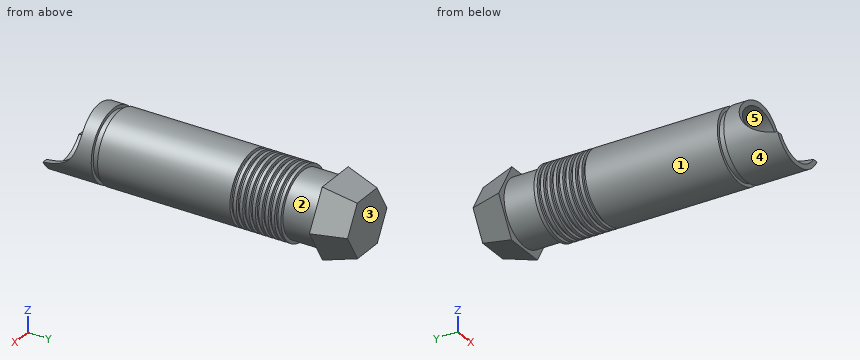
```python
from build123d import *

# Parameters (mm, degrees)
BOSS_EXTRUDE2_DEPTH     = 20
BOSS_EXTRUDE2_TAPER     = 15
BOSS_EXTRUDE3_START     = 30
SKETCH5_R               = 22.3
SKETCH5_R_2             = 19.3
BOSS_EXTRUDE3_DEPTH     = 30
CUT_EXTRUDE1_DEPTH      = 30
CUT_EXTRUDE1_DEPTH_BACK = 30


with BuildPart() as part:
    # Sketch2 → Revolve1 (revolve)
    with BuildSketch(Plane.XY, mode=Mode.PRIVATE) as revolve1_sk:
        Polygon((-19.3, 0), (-19.3, 140), (0, 140), (0, 141), (-20.3, 141), (-20.3, 140), (-20.3, 121), (-22.3, 121), (-22.3, 119), (-20.3, 119), (-20.3, 117), (-22.3, 117), (-22.3, 115), (-20.3, 115), (-20.3, 113), (-22.3, 113), (-22.3, 111), (-20.3, 111), (-20.3, 109), (-22.3, 109), (-22.3, 107), (-20.3, 107), (-20.3, 105), (-22.3, 105), (-22.3, 103), (-20.3, 103), (-20.3, 101), (-22.3, 101), (-22.3, 99), (-20.3, 99), (-20.3, 97), (-22.3, 97), (-22.3, 95), (-20.3, 95), (-20.3, 93), (-22.3, 93), (-22.3, 91), (-20.3, 91), (-20.3, 89), (-22.3, 89), (-22.3, 6), (-20.3, 6), (-20.3, 2), (-22.3, 2), (-22.3, 0), (-20.3, 0), align=None)
    revolve(revolve1_sk.sketch.rotate(Axis((0, 0, 0), (0, 1, 0)), 270), axis=Axis((0, 0, 0), (0, 1, 0)))

    # Sketch3 → Boss-Extrude2 (add)
    with BuildSketch(Plane(origin=(0, 141, 0), x_dir=(1, 0, 0), z_dir=(0, 1, 0))):
        Polygon((12.685608816, 22.368412154), (-13.02880876, 22.170265574), (-25.714417576, -0.19814658), (-12.685608816, -22.368412154), (13.02880876, -22.170265574), (25.714417576, 0.19814658), align=None)
    extrude(amount=BOSS_EXTRUDE2_DEPTH, taper=BOSS_EXTRUDE2_TAPER)

    # Sketch5 → Boss-Extrude3 (add)
    with BuildSketch(Plane.XZ.offset(BOSS_EXTRUDE3_START)):
        with Locations(Location((0, 0, 0), (0, 0, 270))):
            Circle(SKETCH5_R)
        with Locations(Location((0, 0, 0), (0, 0, 270))):
            Circle(SKETCH5_R_2, mode=Mode.SUBTRACT)
    extrude(amount=-BOSS_EXTRUDE3_DEPTH)

    # Sketch6 → Cut-Extrude1 (cut, two sides: drawn at the far end of the back side and taken through both)
    with BuildSketch(Plane(origin=(0, 0, 0), x_dir=(0, 0, -1), z_dir=(1, 0, 0)).offset(-CUT_EXTRUDE1_DEPTH_BACK)):
        with BuildLine():
            add(Edge.make_bspline(
                [(-29.514134147, -8.8446486), (10.566504281, 2.828326519), (11.451543422, -38.297473123)],
                knots=[0, 0, 0, 1, 1, 1], degree=2))
            add(Edge.make_bspline(
                [(-29.514134147, -8.8446486), (-38.265876715, -53.637701487), (11.451543422, -38.297473123)],
                knots=[0, 0, 0, 1, 1, 1], degree=2))
        make_face()
    extrude(amount=CUT_EXTRUDE1_DEPTH + CUT_EXTRUDE1_DEPTH_BACK, mode=Mode.SUBTRACT)


solid = part.part
```
CAD build for the part. Positions are in the model's coordinates, mm. Face numbers are marked on the shaded views. A direction names the side the tool comes from. Coordinates: 2 decimals unless noted, no trailing zeros. Loops run counter-clockwise (first coordinate to the right, second up) from the corner with the lowest first, then second, coordinate; pieces in that order, holes last. Notation, with made-up numbers: (-28, 5) - (-1, 5) arc R18 ccw to (-1, 13) - close; hole circle Ø9 at (85.25, 45.25). An arc over 180 degrees is marked (long way). Return JSON: item names as keys, results as strings.
1. Band-saw the part on A-A (y = 73). Give the cut face in (x, z).
Result:
{"outline": "circle Ø44.6 at (0, 0); hole circle Ø38.6 at (0, 0)"}
2. Mould opens along X. For the marked faces 3, 4 and 5 say: released by +X, released by -X, zero draft, split by the parting line, or undercut.
Result:
{"face 3": "zero draft", "face 4": "split by the parting line", "face 5": "undercut"}
3. Drop flat-ended pins along their axis: pin 1 (1.5 mm diameter, centred on y = 136, z = -3.5, fed in from +X); pin 2 (13.5 mm diameter, centred on x = -8, z = 10, fed in from -Y); pin 3 (12 mm diameter, centred on y = 19, z = -9, fed in from -X). Give the stop position or say it passes through.
Result:
{"pin 1": "stops at x = 20.11", "pin 2": "stops at y = -6.35", "pin 3": "stops at x = -22.1"}
4. 3-axis set-ups, long thin cutter, end or side, ignore diameter. For the marked faces 1 and 2: which of +Z, -Z, +X, -X, +Y, -Y reach the whole face in a straight line?
Result:
{"face 1": "-Y", "face 2": "none"}
5. Probe L1, parallel to X at y = 55.5, z = 0; L2, parallel to Z at x = 0.5, y = 72; L3, parallel to Y at x = -2, z = 8. List the from-to ranges inside material, lowest first. Write a range as from..to.
Result:
{"L1": "x = -22.3..-19.3, 19.3..22.3", "L2": "z = -22.29..-19.29, 19.29..22.29", "L3": "y = 140..161"}
